Answer from the drawing. Dimensions are ordinates in mm from the lowest x, y and z of the part. A direction names the side the tool comes from. Round coordinates to 2 decimals unless told otherwise and drop trailing zeros. Order: outer loops, then holes, each group sorted by start corner. A loop starts at its lowest first (then second) coordinate and runs counter-clockwise, first axis right, second up.
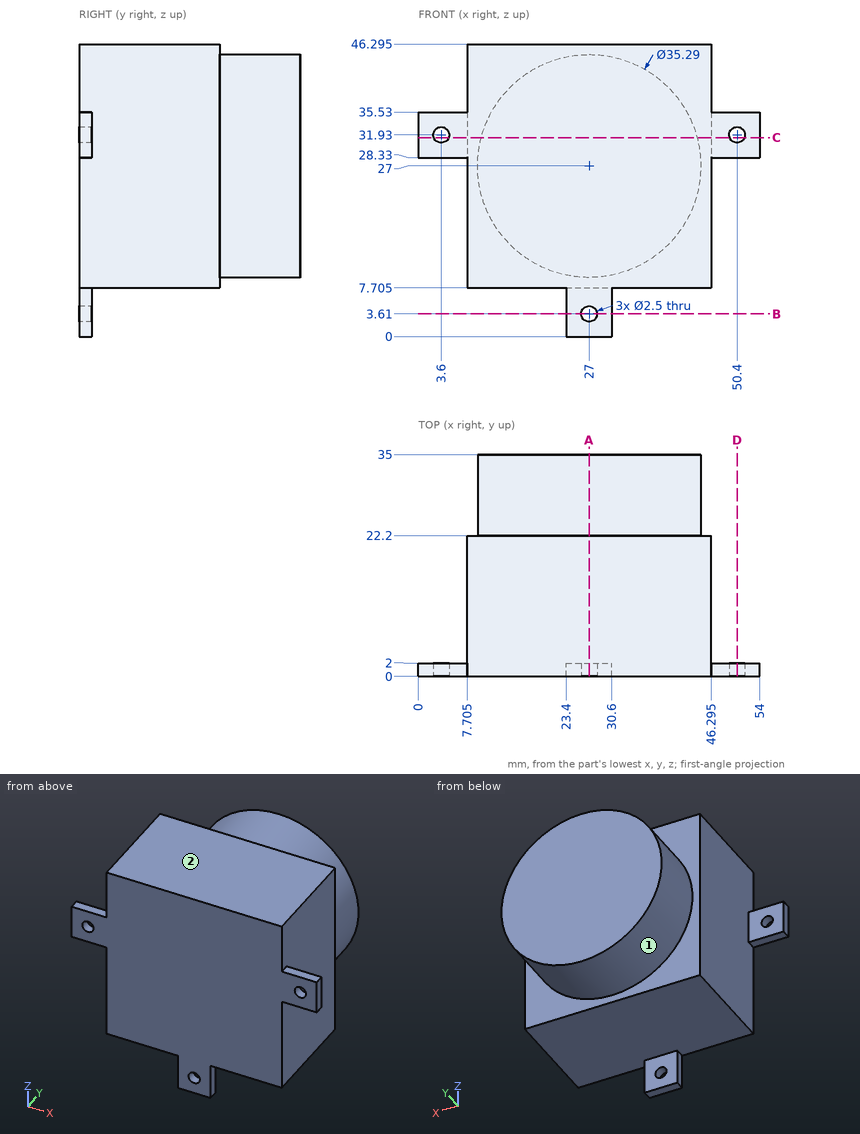
Q1. A cutting plane is placed at A-A, the plane x = 27. Give the vertices of the cut face in (y, z) (3 decimals), plus the area to 3 significant figures.
Outcome:
outline: (0, 0) - (2, 0) - (2, 2.36) - (0, 2.36) - close; (0, 4.86) - (2, 4.86) - (2, 7.705) - (22.2, 7.705) - (22.2, 9.355) - (35, 9.355) - (35, 44.645) - (22.2, 44.645) - (22.2, 46.295) - (0, 46.295) - close
area: 1,320 mm2
Q2. Flat-ended cylindrical pins translate along their axes: pin 1 (1.5 mm diameter, centred on y = 20, z = 19, fed in from -X) (3 decimals); pin 2 (5 mm diameter, centred on x = 48, z = 19, fed in from +Y); pin 3 (2 mm diameter, centred on y = 1.5, z = 5.5, fed in from +X). Find the tip coordinate at first contact, or state that the pin passes through.
Outcome:
pin 1: stops at x = 7.705
pin 2: stops at y = 22.2
pin 3: stops at x = 30.6
Q3. A cutting plane is placed at C-C, the plane z = 31.5. Give the vertices of the cut face in (x, y) (3 decimals).
Outcome:
outline: (0, 0) - (2.426, 0) - (2.426, 2) - (0, 2) - close; (4.774, 0) - (49.226, 0) - (49.226, 2) - (46.295, 2) - (46.295, 22.2) - (44.062, 22.2) - (44.062, 35) - (9.938, 35) - (9.938, 22.2) - (7.705, 22.2) - (7.705, 2) - (4.774, 2) - close; (51.574, 0) - (54, 0) - (54, 2) - (51.574, 2) - close
Q4. A cutting plane is placed at D-D, the plane x = 50.4. Give the vertices of the cut face in (y, z).
Outcome:
outline: (0, 28.33) - (2, 28.33) - (2, 30.68) - (0, 30.68) - close; (0, 33.18) - (2, 33.18) - (2, 35.53) - (0, 35.53) - close
Q5. A cutting plane is placed at B-B, the plane z = 3.61. Give the vertices of the cut face in (x, y).
Outcome:
outline: (23.4, 0) - (25.75, 0) - (25.75, 2) - (23.4, 2) - close; (28.25, 0) - (30.6, 0) - (30.6, 2) - (28.25, 2) - close
Q6. Straight lines are drawn through the part: probe 1 along X at (y, z) = (1.3, 31.93); probe 2 along Z at (x, y) = (35, 13.5) (3 decimals); probe 3 along Y at (x, z) = (36, 9.5). For each, find the intervals that lie inside material, in ascending order.
Outcome:
probe 1: x = 0 to 2.35, 4.85 to 49.15, 51.65 to 54
probe 2: z = 7.705 to 46.295
probe 3: y = 0 to 22.2
Q7. For the marked faces 1 and 2, determine the directions among +Z, -Z, +X, -X, +Y, -Y from which every point of the face is accessible in a straight line to the end or side of a thin tool.
Outcome:
face 1: +Y
face 2: +Z, +X, -X, +Y, -Y
